```python
from build123d import *

# Parameters (mm, degrees)
ESQUISSE1_W             = 70
ESQUISSE1_H             = 42
BOSS_EXTRU_1_DEPTH      = 2
D_GAGEMENT_M41_D        = 4.5
ESQUISSE4_R             = 5.5
ENL_V_MAT_EXTRU_1_DEPTH = 3
ESQUISSE2_R             = 1.5
ENL_V_MAT_EXTRU_2_DEPTH = 3


with BuildPart() as part:
    # Esquisse1 → Boss.-Extru.1 (new body)
    with BuildSketch(Plane.XY):
        with Locations((35, 21)):
            Rectangle(ESQUISSE1_W, ESQUISSE1_H)
    extrude(amount=BOSS_EXTRU_1_DEPTH)

    # Dégagement M41 (through all)
    with Locations(Plane(origin=(35, 32.5, 0), x_dir=(-1, 0, 0), z_dir=(0, 0, -1))):
        with Locations((0, 0), (-12.5, -12.5), (0, -25), (12.5, -12.5)):
            Hole(D_GAGEMENT_M41_D / 2)

    # Esquisse4 → Enlèv. mat.-Extru.1 (cut, through all)
    with BuildSketch(Plane(origin=(0, 0, 0), x_dir=(-1, 0, 0), z_dir=(0, 0, -1))):
        with Locations((-35, 20)):
            Circle(ESQUISSE4_R)
    extrude(amount=-ENL_V_MAT_EXTRU_1_DEPTH, mode=Mode.SUBTRACT)

    # Esquisse2 → Enlèv. mat.-Extru.2 (cut, through all)
    with BuildSketch(Plane(origin=(0, 0, 0), x_dir=(-1, 0, 0), z_dir=(0, 0, -1))):
        with Locations((-9.5, 20)):
            Circle(ESQUISSE2_R)
    extrude(amount=-ENL_V_MAT_EXTRU_2_DEPTH, mode=Mode.SUBTRACT)


solid = part.part
```
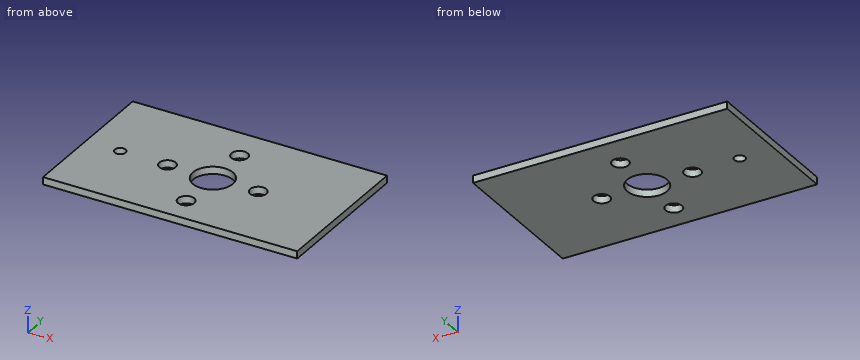
Here's how the part is built. I have some questions about the finished solid (model axes, mm). Round coordinates to 2 decimals unless told otherwise and drop trailing zeros. Write each loop counter-clockwise with the first axis right and the second up, starting at its lowest first coordinate (ties: lowest second). Pieces come first, ordered by that corner, then holes. Notation, with made-up numbers: M -39.5,67 L -14.5,67 A28 ccw -14.5,87 Z; hole C 8,68.5 d7. An arc over 180 degrees is marked long. Answer as CSV lines item,"result". Start each with the question number.
1. Suppose I cut it at C-C on y = 7.5. Write out the boundary of the cut face in (x, z), then the cut area to 3 significant figures.
2. Suppose I cut it at D-D on x = 22.5. Write out the boundary of the cut face in (y, z).
3. Suppose I cut it at B-B on z = 0.75. Write out the boundary of the cut face in (x, y), then the cut area to 3 significant figures.
4. I need wall thicknesses on probe 1 along Y at (x, z) = (35, 0.5); probe 2 along Y at (x, z) = (47.5, 1.5); probe 3 along X at (y, z) = (19, 0.2). Which ranges of each line are inside material? Lowest first, please.
5. Suppose I cut it at A-A on x = 35. Write out the boundary of the cut face in (y, z).
6. I'm going to push a flat-ended pin straight in: pin 1 Ø2.5 at (x, y) = (22.5, 20) entering from -Z. Where does the tip first touch, or does it pass through?
Check result:
1,outline,"M 0,0 L 32.75,0 L 32.75,2 L 0,2 Z; M 37.25,0 L 70,0 L 70,2 L 37.25,2 Z"
1,area,"131 mm2"
2,outline,"M 0,0 L 17.75,0 L 17.75,2 L 0,2 Z; M 22.25,0 L 42,0 L 42,2 L 22.25,2 Z"
3,outline,"M 0,0 L 70,0 L 70,42 L 0,42 Z; hole C 9.5,20 d3; hole C 22.5,20 d4.5; hole C 35,20 d11; hole C 35,7.5 d4.5; hole C 35,32.5 d4.5; hole C 47.5,20 d4.5"
3,area,"2,770 mm2"
4,probe 1,"y = 0 to 5.25, 9.75 to 14.5, 25.5 to 30.25, 34.75 to 42"
4,probe 2,"y = 0 to 17.75, 22.25 to 42"
4,probe 3,"x = 0 to 8.38, 10.62 to 20.48, 24.52 to 29.59, 40.41 to 45.48, 49.52 to 70"
5,outline,"M 0,0 L 5.25,0 L 5.25,2 L 0,2 Z; M 9.75,0 L 14.5,0 L 14.5,2 L 9.75,2 Z; M 25.5,0 L 30.25,0 L 30.25,2 L 25.5,2 Z; M 34.75,0 L 42,0 L 42,2 L 34.75,2 Z"
6,pin 1,"passes through"
